from build123d import *

# Parameters (mm, degrees)
F1_DEPTH = 15
F2_W     = 13.3
F2_H     = 13.3
F3_DEPTH = 26


with BuildPart() as f1:
    # F0 (on Top) → F1 (new body)
    with BuildSketch(Plane.XY):
        with BuildLine():
            Line((8.68, -5.582114), (8.68, 5.582114))
            ThreePointArc((8.68, 5.582114), (-10.32, 0), (8.68, -5.582114))
        make_face()
    extrude(amount=F1_DEPTH)

    # F2 (on face) → F3 (join)
    with BuildSketch(Plane.XY.offset(15)):
        Rectangle(F2_W, F2_H)
    extrude(amount=F3_DEPTH)


solid = f1.part
Geometry check sheet. Reference: the model listing, model coordinates, mm. A direction names the side the tool comes from. Coordinates: 2 decimals unless noted, no trailing zeros. Order: outer loops, then holes, each group sorted by start corner. A loop starts at its lowest first (then second) coordinate and runs counter-clockwise, first axis right, second up. Notation, with made-up numbers: (-36, 41) - (-7, 41) arc R18 cw to (-7, 59) - close; hole circle Ø10 at (60, 14). An arc over 180 degrees is marked (long way). Answer in a Markdown table with one row per item. Add a question column.
1) Gauge pin test, flat ends, axial feed: P1, Ø1.5, axis at x = -8, y = -4.5, coming from the +Z side; P2, Ø4, axis at x = 1, z = 24, coming from the -Y side; P3, Ø5, axis at x = -5.5, z = 23, coming from the +Y side. Record the tip position at first contact, or that the pin passes through.
2) Set-up check for faces 1 (the flat face through (0, -6.65, 28)), 2 (the flat face through (0, 0, 41)), 3 (the flat face through (-6.65, 0, 28)), 4 (the flat face through (0, 6.65, 28)), 5 (the flat face through (6.65, 0, 28)): record each of +Z, -Z, +X, -X, +Y, -Y from which the full face is reachable in a straight line by a thin tool's end or side.
3) Cross-section at B-B, the plane x = 0. Record the cut outline in (y, z).
4) Cross-section at D-D, the plane x = -8.25. Record the cut outline in (y, z), then the cut area to 3 significant figures.
5) Material ranges on line 1 along Y through (x, z) = (5, 22); line 2 along Z through (x, y) = (4.75, -7.5), recorded low to high. Write a range as [from, to].
6) Cross-section at C-C, the plane z = 11.5. Record the cut outline in (x, y).
7) Cross-section at A-A, the plane y = 0. Record the cut outline in (x, z), then the cut area to 3 significant figures.
Check result:
| question | item | result |
|---|---|---|
| 1 | P1 | stops at z = 15 |
| 1 | P2 | stops at y = -6.65 |
| 1 | P3 | stops at y = 6.65 |
| 2 | face 1 | +Z, +X, -X, -Y |
| 2 | face 2 | +Z, +X, -X, +Y, -Y |
| 2 | face 3 | +Z, -X, +Y, -Y |
| 2 | face 4 | +Z, +X, -X, +Y |
| 2 | face 5 | +Z, +X, +Y, -Y |
| 3 | outline | (-10.32, 0) - (10.32, 0) - (10.32, 15) - (6.65, 15) - (6.65, 41) - (-6.65, 41) - (-6.65, 15) - (-10.32, 15) - close |
| 4 | outline | (-6.2, 0) - (6.2, 0) - (6.2, 15) - (-6.2, 15) - close |
| 4 | area | 186 mm² |
| 5 | line 1 | y = [-6.65, 6.65] |
| 5 | line 2 | z = [0, 15] |
| 6 | outline | (8.68, -5.58) - (8.68, 5.58) arc R10.32 ccw (long way) to start |
| 7 | outline | (-10.32, 0) - (8.68, 0) - (8.68, 15) - (6.65, 15) - (6.65, 41) - (-6.65, 41) - (-6.65, 15) - (-10.32, 15) - close |
| 7 | area | 631 mm² |
